Study the drawing (mm; zero at the part's minimum x, y, z) and answer. A direction names the side the tool comes from. Give positions to 0.01 mm unless a question says otherwise; leave off trailing zeros. Loops run counter-clockwise (first coordinate to the right, second up) from the corner with the lowest first, then second, coordinate; pieces in that order, holes last. Notation, with made-up numbers: M 1,84.5 L 17,84.5 A19 cw 17,109.5 Z; hole C 11,-24.75 d11. An arc over 180 degrees is marked long. Return JSON: item names as keys, results as strings.
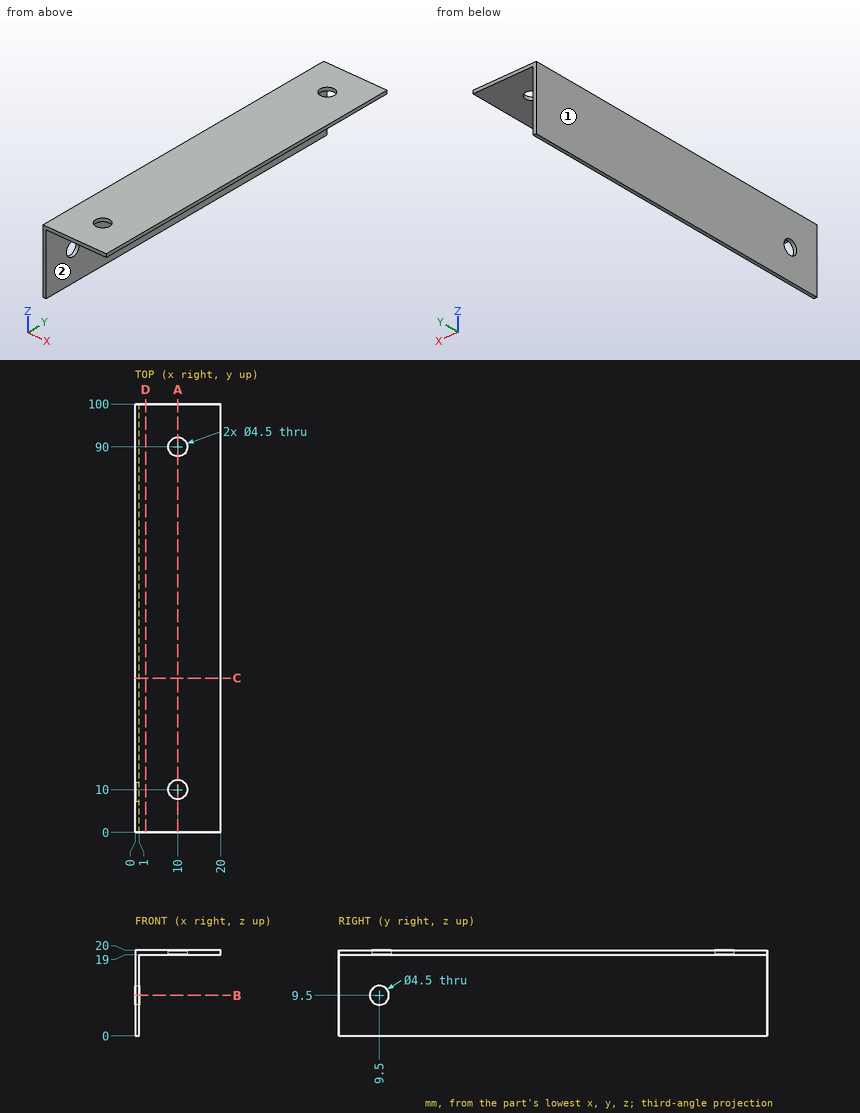
(1) The part is cut by section D-D (x = 2.5). Determine the outline of the cut face in (y, z), and give its area (3 significant figures).
Values follow:
{"outline": "M 0,19 L 100,19 L 100,20 L 0,20 Z", "area": "100 mm²"}
(2) Given pin 1 (4 mm diameter, centred on y = 78.5, z = 6.5, fed in from +X); pin 2 (5.5 mm diameter, centred on x = 10.5, y = 45, fed in from -Z); pin 3 (2.5 mm diameter, centred on x = 10, y = 90, fed in from -Z), each flat-ended and moving along its own axis, determine where each tip first touches the part or whether it passes through.
Values follow:
{"pin 1": "x = 1", "pin 2": "z = 19", "pin 3": "through"}
(3) A tool of negligible diameter and unlimited length cuts with its end or side. For the marked faces 1 and 2, from which of +Z, -Z, +X, -X, +Y, -Y can it reach the whole face along a straight path? Write none if from no direction.
Values follow:
{"face 1": "+Z, -Z, -X, +Y, -Y", "face 2": "-Z, +X, +Y, -Y"}
(4) The part is cut by section B-B (z = 9.5). Determine the outline of the cut face in (x, y).
Values follow:
{"outline": "M 0,0 L 1,0 L 1,7.25 L 0,7.25 Z; M 0,11.75 L 1,11.75 L 1,100 L 0,100 Z"}
(5) The part is cut by section A-A (x = 10). Determine the outline of the cut face in (y, z), and give its area (3 significant figures).
Values follow:
{"outline": "M 0,19 L 7.75,19 L 7.75,20 L 0,20 Z; M 12.25,19 L 87.75,19 L 87.75,20 L 12.25,20 Z; M 92.25,19 L 100,19 L 100,20 L 92.25,20 Z", "area": "91.0 mm²"}
(6) Straight lines are drawn through the part: line 1 along Y through (x, z) = (10, 19.25); line 2 along Y through (x, z) = (0.5, 9.5); line 3 along X through (y, z) = (80.5, 17.75). For each, find the intervals that lie inside material, in ascending order.
Values follow:
{"line 1": "0 to 7.75, 12.25 to 87.75, 92.25 to 100", "line 2": "0 to 7.25, 11.75 to 100", "line 3": "0 to 1"}
(7) The part is cut by section C-C (y = 36). Determine the outline of the cut face in (x, z).
Values follow:
{"outline": "M 0,0 L 1,0 L 1,19 L 20,19 L 20,20 L 0,20 Z"}
